```python
from build123d import *

# Parameters (mm, degrees)
BASE_FLANGE1_DEPTH           = 406.4
CUT_EXTRUDE1_DEPTH           = 416.864403983
F_1_4_CLEARANCE_HOLE1_D      = 6.858
F_10_0_1935_DIAMETER_HOLE1_D = 4.9149
SKETCH15_W                   = 10.69848
SKETCH15_H                   = 17.546986719
CUT_EXTRUDE4_DEPTH           = 411.595144272
SKETCH16_W                   = 44.45
SKETCH16_H                   = 17.546986719
CUT_EXTRUDE5_DEPTH           = 411.595144272
FILLET2_R                    = 1.27
F_1_2_0_5_DIAMETER_HOLE1_D   = 12.7
SKETCH19_W                   = 38.1
SKETCH19_H                   = 22.225
CUT_EXTRUDE6_DEPTH           = 5.76326
F_7_8_0_875_DIAMETER_HOLE1_D = 22.225
FILLET3_R                    = 2.54


# Sheet-metal steps are written as plain solids
with BuildPart() as part:
    # Sketch1 → Base-Flange1 (new body)
    with BuildSketch(Plane.XY):
        with BuildLine():
            Line((38.1, -44.45), (38.1, -5.76326))
            ThreePointArc((38.1, -5.76326), (36.411980228, -1.688019772), (32.33674, 0))
            Line((32.33674, 0), (-32.33674, 0))
            ThreePointArc((-32.33674, 0), (-36.411980228, -1.688019772), (-38.1, -5.76326))
            Line((-38.1, -5.76326), (-38.1, -44.45))
            Line((-38.1, -44.45), (-35.51174, -44.45))
            Line((-35.51174, -44.45), (-35.51174, -5.76326))
            ThreePointArc((-35.51174, -5.76326), (-34.58180403, -3.51819597), (-32.33674, -2.58826))
            Line((-32.33674, -2.58826), (32.33674, -2.58826))
            ThreePointArc((32.33674, -2.58826), (34.58180403, -3.51819597), (35.51174, -5.76326))
            Line((35.51174, -5.76326), (35.51174, -44.45))
            Line((35.51174, -44.45), (38.1, -44.45))
        make_face()
    extrude(amount=BASE_FLANGE1_DEPTH)

    # Sketch7 → Cut-Extrude1 (cut, through all)
    with BuildSketch(Plane(origin=(38.1, 0, 0), x_dir=(0, 0, -1), z_dir=(1, 0, 0))):
        Polygon((-406.4, -16.515725506), (-378.120513741, -8.93826), (-366.271252427, -8.93826), (-366.271252427, 0), (-406.4, 0), align=None)
        Polygon((0, 0), (0, -16.515725506), (-28.279486259, -8.93826), (-40.128747573, -8.93826), (-40.128747573, 0), align=None)
    extrude(amount=-CUT_EXTRUDE1_DEPTH, mode=Mode.SUBTRACT)

    # 1/4 Clearance Hole1 (through all)
    with Locations(Plane(origin=(0, 0, 0), x_dir=(1, 0, 0), z_dir=(0, 1, 0))):
        with Locations((0, -104.14), (0, -72.39)):
            Hole(F_1_4_CLEARANCE_HOLE1_D / 2)

    # #10 (0.1935) Diameter Hole1 (through all)
    with Locations(Plane.ZY.offset(38.1)):
        with Locations((9.525, -34.925), (9.525, -21.59), (31.75, -34.925), (31.75, -15.875), (374.65, -15.875), (374.65, -34.925), (396.875, -21.59), (396.875, -34.925), (155.575, -13.97), (155.575, -34.925), (250.825, -34.925), (250.825, -13.97)):
            Hole(F_10_0_1935_DIAMETER_HOLE1_D / 2)

    # Sketch15 → Cut-Extrude4 (cut, through all)
    with BuildSketch(Plane(origin=(0, 0, 0), x_dir=(1, 0, 0), z_dir=(0, 1, 0))):
        with Locations((26.9875, -130.37599336)):
            Rectangle(SKETCH15_W, SKETCH15_H)
        with Locations((-26.9875, -130.37599336)):
            Rectangle(SKETCH15_W, SKETCH15_H)
    extrude(amount=-CUT_EXTRUDE4_DEPTH, mode=Mode.SUBTRACT)

    # Sketch16 → Cut-Extrude5 (cut, through all)
    with BuildSketch(Plane(origin=(0, 0, 0), x_dir=(1, 0, 0), z_dir=(0, 1, 0))):
        with Locations((0, -276.024006641)):
            Rectangle(SKETCH16_W, SKETCH16_H)
    extrude(amount=-CUT_EXTRUDE5_DEPTH, mode=Mode.SUBTRACT)

    # Fillet2
    fillet2_edges = [part.edges().sort_by_distance(p)[0] for p in [
        (21.63826, -1.29413, 139.149486719),
        (21.63826, -1.29413, 121.6025),
        (32.33674, -1.29413, 121.6025),
        (32.33674, -1.29413, 139.149486719),
        (-32.33674, -1.29413, 121.6025),
        (-21.63826, -1.29413, 121.6025),
        (-21.63826, -1.29413, 139.149486719),
        (-32.33674, -1.29413, 139.149486719),
        (-22.225, -1.29413, 284.7975),
        (-22.225, -1.29413, 267.250513281),
        (22.225, -1.29413, 267.250513281),
        (22.225, -1.29413, 284.7975),
    ]]
    fillet(fillet2_edges, radius=FILLET2_R)

    # 1/2 (0.5) Diameter Hole1 (through all)
    with Locations(Plane.ZY.offset(38.1)):
        with Locations((171.45, -23.607014), (234.95, -23.607014)):
            Hole(F_1_2_0_5_DIAMETER_HOLE1_D / 2)

    # Sketch19 → Cut-Extrude6 (cut)
    with BuildSketch(Plane.ZY.offset(38.1)):
        with Locations((86.6775, -11.1125)):
            Rectangle(SKETCH19_W, SKETCH19_H)
    extrude(amount=-CUT_EXTRUDE6_DEPTH, mode=Mode.SUBTRACT)

    # 7/8 (0.875) Diameter Hole1 (through all)
    with Locations(Plane(origin=(0, 0, 0), x_dir=(1, 0, 0), z_dir=(0, 1, 0))):
        with Locations((0, -238.252), (0, -206.502)):
            Hole(F_7_8_0_875_DIAMETER_HOLE1_D / 2)

    # Fillet3
    fillet3_edges = [part.edges().sort_by_distance(p)[0] for p in [
        (36.80587, -16.515725506, 0),
        (-36.80587, -16.515725506, 0),
        (36.80587, -44.45, 0),
        (-36.80587, -44.45, 0),
        (36.80587, -44.45, 406.4),
        (-36.80587, -22.225, 67.6275),
        (-36.80587, -22.225, 105.7275),
        (-36.80587, -16.515725506, 406.4),
        (36.80587, -16.515725506, 406.4),
        (-36.80587, -44.45, 406.4),
    ]]
    fillet(fillet3_edges, radius=FILLET3_R)


solid = part.part
```
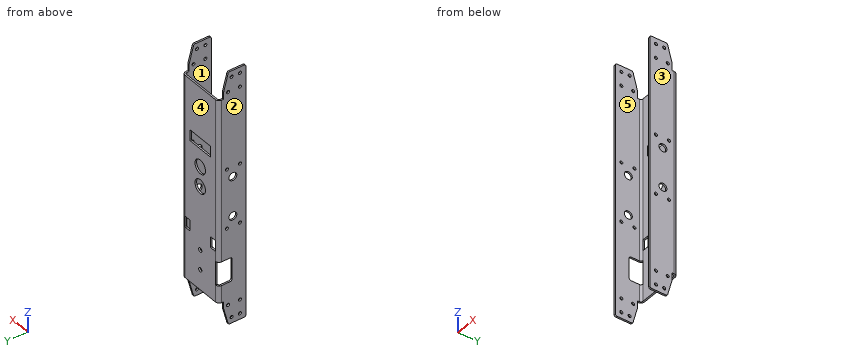
Here's how the part is built. I have some questions about the finished solid (model axes, mm). Face numbers are marked on the shaded views. A direction names the side the tool comes from. Coordinates: 2 decimals unless noted, no trailing zeros. Order: outer loops, then holes, each group sorted by start corner. A loop starts at its lowest first (then second) coordinate and runs counter-clockwise, first axis right, second up.
1) I need wall thicknesses on line 1 (X direction, y = -40, z = 389); line 2 (Y direction, x = 37, z = 31); line 3 (X direction, y = -5, z = 349.5). Which ranges of each line are inside material? Lowest first, please.
2) Imagine slicing it at A-A on z = 58.5. List the corners of the cut face in (x, y) for me (3 decimals).
3) Which directions (+Z, -Z, +X, -X, +Y, -Y) give clear straight access to the entire face, cutting with the end or side of a thin tool? Please do the marked faces 4 and 5.
4) Will these pins go through, and if not, where does the flat tip stop? pin 1 (12 mm diameter, centred on x = -28, z = 116.5, fed in from -Y); pin 2 (12 mm diameter, centred on x = -17.5, z = 88, fed in from -Y); pin 3 (1.3 mm diameter, centred on x = -1, y = -1.5, fed in from -Z); pin 4 (3 mm diameter, centred on y = -34.925, z = 155.575, fed in from +X).
5) We'd pull the mould along X, two halves only. Please class the marked faces 1, 2 and 3: +X half, -X half, draft (parallel to the pull), parting line (faces both ways), or undercut.
Response values:
1. line 1: x = -38.1 to -35.51, 35.51 to 38.1
1. line 2: y = -44.45 to -37.27, -32.58 to -18.22, -13.53 to -8.94
1. line 3: x = -38.05 to -35.42, 35.42 to 38.05
2. outline: (-38.1, -44.45) - (-35.512, -44.45) - (-35.512, -5.763) arc R3.175 cw to (-32.337, -2.588) - (32.337, -2.588) arc R3.175 cw to (35.512, -5.763) - (35.512, -44.45) - (38.1, -44.45) - (38.1, -5.763) arc R5.763 ccw to (32.337, 0) - (-32.337, 0) arc R5.763 ccw to (-38.1, -5.763) - close
3. face 4: +Z, -Z, +X, -X, +Y
3. face 5: +Z, -Z, -Y
4. pin 1: stops at y = -3.06
4. pin 2: stops at y = -2.59
4. pin 3: stops at z = 40.13
4. pin 4: passes through
5. face 1: undercut
5. face 2: -X half
5. face 3: +X half
